The drawing under review shows one solid part. Ordinate dimensions are in mm from its lowest x, y, z. A direction names the side the tool comes from. Coordinates: 2 decimals unless noted, no trailing zeros. Order: outer loops, then holes, each group sorted by start corner. A loop starts at its lowest first (then second) coordinate and runs counter-clockwise, first axis right, second up.
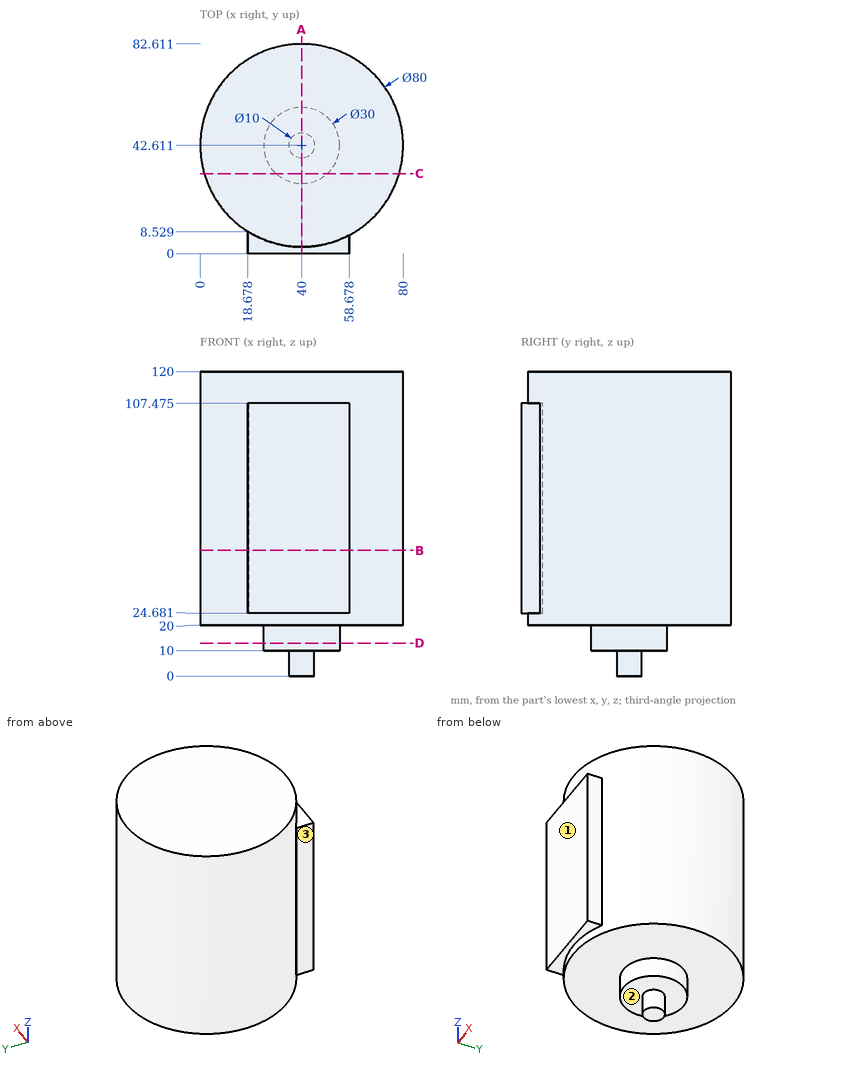
(1) We need section B-B, the plane z = 49.5. Write out the cut boundary in (x, y).
A:
outline: (18.68, 0) - (58.68, 0) - (58.68, 7.24) arc R40 ccw (long way) to (19.06, 8.53) - (18.68, 8.53) - close
(2) We need section C-C, the plane y = 31.5. Write out the cut boundary in (x, z).
A:
outline: (1.57, 20) - (29.92, 20) - (29.92, 10) - (50.08, 10) - (50.08, 20) - (78.43, 20) - (78.43, 120) - (1.57, 120) - close
(3) Wall thickness on probe 1 along Y at (x, z) = (40, 54); probe 2 along Z at (x, y) = (14.5, 51.5); probe 3 along Z at (x, y) = (37.5, 57): over which ranges is each line inside the solid? List them lowest first.
A:
probe 1: y = 0 to 82.61
probe 2: z = 20 to 120
probe 3: z = 10 to 120
(4) We need section D-D, the plane z = 13. Write out the cut boundary in (x, y), and give its area (3 significant figures).
A:
outline: circle Ø30 at (40, 42.61)
area: 707 mm2
(5) We need section A-A, the plane x = 40. Write out the cut boundary in (y, z) (1 decimal).
A:
outline: (0, 24.7) - (2.6, 24.7) - (2.6, 20) - (27.6, 20) - (27.6, 10) - (37.6, 10) - (37.6, 0) - (47.6, 0) - (47.6, 10) - (57.6, 10) - (57.6, 20) - (82.6, 20) - (82.6, 120) - (2.6, 120) - (2.6, 107.5) - (0, 107.5) - close
(6) For pin 1 Ø3 at (y, z) = (24, 59) entering from -X (1 decimal); pin 2 Ø8 at (x, z) = (60, 90) entering from +Y; pin 3 Ø24 at (x, y) = (44, 62) entering from -Z, all flat-tipped, find the tip position at first contact; note any pin that passes through.
A:
pin 1: stops at x = 3.8
pin 2: stops at y = 79.27
pin 3: stops at z = 10
(7) Machinability: for the marked faces 1, 2 and 3, which of the approach directions +Z, -Z, +X, -X, +Y, -Y give a long, thin tool a straight path to every point of the face, cutting with its end or side? Answer none if there is none.
A:
face 1: +Z, -Z, +X, -X, -Y
face 2: -Z
face 3: +Z, -Z, -X, -Y
